```python
from build123d import *

# Parameters (mm, degrees)
F0_W      = 18.2
F0_H      = 13
F1_DEPTH  = 11.3
F2_R      = 4
F2_R_2    = 3
F3_DEPTH  = 1
F3_FACE_R = 3
F4_DEPTH  = 10
F5_W      = 2
F5_H      = 0.75
F6_DEPTH  = 3.8


with BuildPart() as f1:
    # F0 (on Top) → F1 (new body)
    with BuildSketch(Plane.XY):
        Rectangle(F0_W, F0_H)
    extrude(amount=F1_DEPTH)

    # F2 (on face) → F3 (join)
    with BuildSketch(Plane.XY.offset(11.3)):
        Circle(F2_R)
        Circle(F2_R_2, mode=Mode.SUBTRACT)
    extrude(amount=F3_DEPTH)

    # F3_face (on face) → F4 (join)
    with BuildSketch(Plane.XY.offset(11.3)):
        Circle(F3_FACE_R)
    extrude(amount=F4_DEPTH)

    # F5 (on face) → F6 (join)
    with BuildSketch(Plane(origin=(0, 0, 0), x_dir=(1, 0, 0), z_dir=(0, 0, -1))):
        with Locations((-5.4, 4.725)):
            Rectangle(F5_W, F5_H)
        with Locations((0, 4.725)):
            Rectangle(F5_W, F5_H)
        with Locations((5.4, 4.725)):
            Rectangle(F5_W, F5_H)
        with Locations((5.4, 0)):
            Rectangle(F5_W, F5_H)
        Rectangle(F5_W, F5_H)
        with Locations((-5.4, 0)):
            Rectangle(F5_W, F5_H)
        with Locations((5.4, -4.725)):
            Rectangle(F5_W, F5_H)
        with Locations((0, -4.725)):
            Rectangle(F5_W, F5_H)
        with Locations((-5.4, -4.725)):
            Rectangle(F5_W, F5_H)
    extrude(amount=F6_DEPTH)


solid = f1.part
```
Input: part model. Units: mm. Frame: model coordinates. A direction names the side the tool comes from. Round coordinates to 2 decimals unless told otherwise and drop trailing zeros. Loops run counter-clockwise (first coordinate to the right, second up) from the corner with the lowest first, then second, coordinate; pieces in that order, holes last. Notation, with made-up numbers: M 67.25,-13.75 L 104.25,-13.75 A33 cw 104.25,17.25 Z; hole C -0.5,75 d2. An arc over 180 degrees is marked long. Answer in a Markdown table with one row per item. Add a question column.
1. Section A-A (z = -2). Give the number of separate pieces and of enclosed holes in the cut face, and give its area (3 significant figures).
2. Mould query, pull axis Y, two halves, no side actions, for faces 4 (the face through (-5, -5.1, -2)), 5 (the face through (-3, 0, 17)), 6 (the face through (5, 4.35, -2)), 7 (the face through (0, 0, 21.3)). Classes: released by +Y, released by -Y, zero draft, split by the parting line, or undercut.
3. Ray query, probe 1 along Z at (x, y) = (-8, -2.25); probe 2 along Z at (x, y) = (-3.25, -1); probe 3 along X at (y, z) = (1.25, 12.75). Return the intervals inside material, ascending.
4. Contact query for flat-ended pins moving along their axis: pin 1 (0.8 mm diameter, centred on y = -4.5, z = -1, fed in from -X); pin 2 (5 mm diameter, centred on y = -3.5, z = 14, fed in from +X); pin 3 (1.6 mm diameter, centred on x = 0, z = -2, fed in from -Y). Output: stop coordinate, or through.
5. Section D-D (z = 18). Output: boundary loops of the cut face in (x, y).
6. Section B-B (x = 5.5). Output: boundary loops of the cut face in (y, z) (3 decimals).
7. Set-up query: faces 1 (the face through (-5, -0.375, -2)), 2 (the face through (-5, 5.1, -2)), 3 (the face through (-0.867, -3.905, 11.793)). Return all of +Z, -Z, +X, -X, +Y, -Y with unobstructed straight access to the full face (end or side cutting, diameter ignored); none if empty.
8. Section C-C (y = 0). Output: boundary loops of the cut face in (x, z).
Values follow:
| question | item | result |
|---|---|---|
| 1 | separate pieces | 9 |
| 1 | enclosed holes | 0 |
| 1 | area | 13.5 mm^2 |
| 2 | face 4 | released by -Y |
| 2 | face 5 | split by the parting line |
| 2 | face 6 | undercut |
| 2 | face 7 | zero draft |
| 3 | probe 1 | 0 to 11.3 |
| 3 | probe 2 | 0 to 12.3 |
| 3 | probe 3 | -2.73 to 2.73 |
| 4 | pin 1 | x = -6.4 |
| 4 | pin 2 | x = 3.64 |
| 4 | pin 3 | y = -5.1 |
| 5 | outline | C 0,0 d6 |
| 6 | outline | M -6.5,0 L -5.1,0 L -5.1,-3.8 L -4.35,-3.8 L -4.35,0 L -0.375,0 L -0.375,-3.8 L 0.375,-3.8 L 0.375,0 L 4.35,0 L 4.35,-3.8 L 5.1,-3.8 L 5.1,0 L 6.5,0 L 6.5,11.3 L -6.5,11.3 Z |
| 7 | face 1 | -Z, +X, -X |
| 7 | face 2 | -Z, +X, -X, +Y |
| 7 | face 3 | +Z |
| 8 | outline | M -9.1,0 L -6.4,0 L -6.4,-3.8 L -4.4,-3.8 L -4.4,0 L -1,0 L -1,-3.8 L 1,-3.8 L 1,0 L 4.4,0 L 4.4,-3.8 L 6.4,-3.8 L 6.4,0 L 9.1,0 L 9.1,11.3 L 4,11.3 L 4,12.3 L 3,12.3 L 3,21.3 L -3,21.3 L -3,12.3 L -4,12.3 L -4,11.3 L -9.1,11.3 Z |
